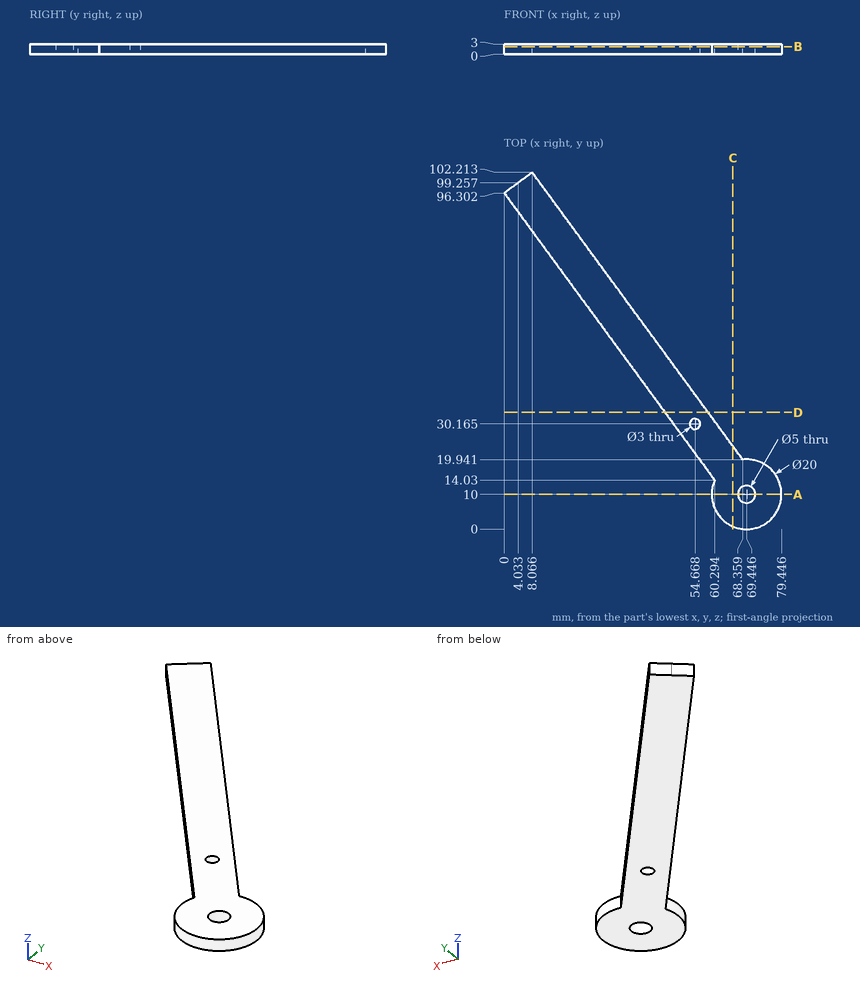
For this review, use the dimensioned drawing (mm, ordinates from the lowest corner) and the shaded views. Round coordinates to 2 decimals unless told otherwise and drop trailing zeros. Order: outer loops, then holes, each group sorted by start corner. A loop starts at its lowest first (then second) coordinate and runs counter-clockwise, first axis right, second up.
1) Consider section B-B (z = 2.25). State the section outline as (x, y) points (1 decimal), plus the area to 3 significant figures.
The answers:
outline: (0, 96.3) - (60.3, 14) arc R10 ccw (long way) to (68.4, 19.9) - (8.1, 102.2) - close; hole circle Ø3 at (54.7, 30.2); hole circle Ø5 at (69.4, 10)
area: 1,300 mm2
2) Consider section D-D (y = 33.5). State the section outline as (x, z) points (1 decimal).
The answers:
outline: (46, 0) - (58.4, 0) - (58.4, 3) - (46, 3) - close
3) Consider section C-C (x = 65.5). State the section outline as (y, z) points.
The answers:
outline: (0.81, 0) - (23.84, 0) - (23.84, 3) - (0.81, 3) - close
4) Consider section A-A (y = 10). State the section outline as (x, z) points (1 decimal).
The answers:
outline: (59.4, 0) - (66.9, 0) - (66.9, 3) - (59.4, 3) - close; (71.9, 0) - (79.4, 0) - (79.4, 3) - (71.9, 3) - close
5) For L1, parallel to X at y = 10, z = 1.2 (1 decimal); L2, parallel to Y at x = 70, z = 2.7 (1 decimal); L3, parallel to Y at x = 48.5, z = 1.4 (1 decimal), list the stretches that pass through material, from the lowest coordinate up.
The answers:
L1: x = 59.4 to 66.9, 71.9 to 79.4
L2: y = 0 to 7.6, 12.4 to 20
L3: y = 30.1 to 47
6) Clearance check with flat-ended pins moving along their axes: pin 1 Ø4 at (x, y) = (69.45, 10) entering from +Z; pin 2 Ø1 at (x, z) = (38, 0.5) entering from -Y; pin 3 Ø8 at (x, y) = (62.5, 30) entering from +Z; pin 4 Ø1.5 at (y, z) = (89, 1.5) entering from -X. State where each tip first meets the part, or that it passes through.
The answers:
pin 1: passes through
pin 2: stops at y = 43.77
pin 3: stops at z = 3
pin 4: stops at x = 4.8
